from build123d import *

# Parameters (mm, degrees)
SKETCH1_R                                    = 12.5
BOSS_EXTRUDE1_DEPTH                          = 1
CUT_EXTRUDE1_REACH                           = 19.706
SKETCH3_R                                    = 4
CSK_FOR_M3_FLAT_COUNTERSUNK_HEAD_SCR_2_COUNT = 2
CSK_FOR_M3_FLAT_COUNTERSUNK_HEAD_SCR_2_PITCH = 14


with BuildPart() as part:
    # Sketch1 → Boss-Extrude1 (new body)
    with BuildSketch(Plane.XY):
        Circle(SKETCH1_R)
    extrude(amount=BOSS_EXTRUDE1_DEPTH)

    # Sketch2 → Cut-Revolve1 (revolve, cut)
    with BuildSketch(Plane(origin=(0, 0, 2), x_dir=(0, 0, 1), z_dir=(-1, 0, 0)), mode=Mode.PRIVATE) as cut_revolve1_sk:
        Polygon((-2, 10), (-1.530086733, 12.665010569), (-2, 12.665010386), align=None)
    revolve(cut_revolve1_sk.sketch.rotate(Axis((0, 0, -0.1), (0, 0, 1)), 270), axis=Axis((0, 0, -0.1), (0, 0, 1)), mode=Mode.SUBTRACT)

    # Sketch3 → Cut-Extrude1 (cut, up to next)
    with BuildSketch(Plane(origin=(0, 0, 0), x_dir=(-1, 0, 0), z_dir=(0, 0, -1)), mode=Mode.PRIVATE) as cut_extrude1_sk1:
        Circle(SKETCH3_R)
    cut_extrude1_tool1 = extrude(cut_extrude1_sk1.sketch, amount=-CUT_EXTRUDE1_REACH, mode=Mode.PRIVATE) & part.part
    add(cut_extrude1_tool1.solids().sort_by_distance((0, 0, 0))[0], mode=Mode.SUBTRACT)

    # Sketch5 → CSK for M3 Flat Countersunk Head Screw1 (revolve, cut)
    with BuildSketch(Plane(origin=(0, 7, 1), x_dir=(0, -1, 0), z_dir=(1, 0, 0))):
        Polygon((0, 0), (0, 1), (1.35, 1), (1.35, 1.15), (2.5, 0), align=None)
    csk_for_m3_flat_countersunk_head_screw1 = revolve(axis=Axis((0, 7, 7.35), (0, 0, -1)), mode=Mode.SUBTRACT)

    # CSK for M3 Flat Countersunk Head Scr 2: CSK for M3 Flat Countersunk Head Screw1 ×2
    with Locations(*[(0, -i * CSK_FOR_M3_FLAT_COUNTERSUNK_HEAD_SCR_2_PITCH, 0) for i in range(1, CSK_FOR_M3_FLAT_COUNTERSUNK_HEAD_SCR_2_COUNT)]):
        add(csk_for_m3_flat_countersunk_head_screw1, mode=Mode.SUBTRACT)


solid = part.part
Source: CAD feature listing. Evaluate the final solid. Frame: model axes, mm. Round coordinates to 2 decimals unless told otherwise and drop trailing zeros. Loops run counter-clockwise (first coordinate to the right, second up) from the corner with the lowest first, then second, coordinate; pieces in that order, holes last. Notation, with made-up numbers: (71, 7.25) - (130, 7.25) arc R11 ccw to (130, 12.25) - close; hole circle Ø4 at (31, -2.75). An arc over 180 degrees is marked (long way). Write item = value, one per line. Start each with the question number.
(1) Section query B-B, the plane y = 0. Output: boundary loops of the cut face in (x, z).
(2) Pin query (flat end, axial travel): pin 1 (7 mm diameter, centred on x = 0, y = 0, fed in from -Z). Return the tip coordinate at first contact, or that it passes through.
(3) Pull-direction query (X, two-part tool) for faces 1 (the face through (-2.202, -9.915, 0.028)), 2 (the face through (-3, 3, 1)), 3 (the face through (0.867, -3.905, 0.493)); classes: +X half, -X half, draft (parallel to the pull), parting line (faces both ways), or undercut.
(4) Section query C-C, the plane z = 0.75. Output: boundary loops of the cut face in (x, y).
(5) Ray query, line 1 along Y through (x, z) = (-0.5, 0.6); line 2 along Y through (x, z) = (0, 0.6); line 3 along X through (y, z) = (6, 0.55). Return the intervals inside material, ascending. Write a range as from..to.
(6) Section query A-A, the plane x = 0. Output: boundary loops of the cut face in (y, z), plus the area to 3 significant figures.
Conclusion:
q1.outline = (-12.5, 0.44) - (-10, 0) - (-4, 0) - (-4, 1) - (-12.5, 1) - close; (4, 0) - (10, 0) - (12.5, 0.44) - (12.5, 1) - (4, 1) - close
q2.pin_1 = through
q3.face_1 = parting line
q3.face_2 = draft
q3.face_3 = undercut
q4.outline = circle Ø25 at (0, 0); hole circle Ø8 at (0, 0); hole circle Ø4.5 at (0, -7); hole circle Ø4.5 at (0, 7)
q5.line_1 = -12.49..-9.04, -4.96..-3.97, 3.97..4.96, 9.04..12.49
q5.line_2 = -12.5..-9.1, -4.9..-4, 4..4.9, 9.1..12.5
q5.line_3 = -10.97..-1.79, 1.79..10.97
q6.outline = (-12.5, 0.44) - (-10, 0) - (-8.5, 0) - (-9.5, 1) - (-12.5, 1) - close; (-5.5, 0) - (-4, 0) - (-4, 1) - (-4.5, 1) - close; (4, 0) - (5.5, 0) - (4.5, 1) - (4, 1) - close; (8.5, 0) - (10, 0) - (12.5, 0.44) - (12.5, 1) - (9.5, 1) - close
q6.area = 7.90 mm2
